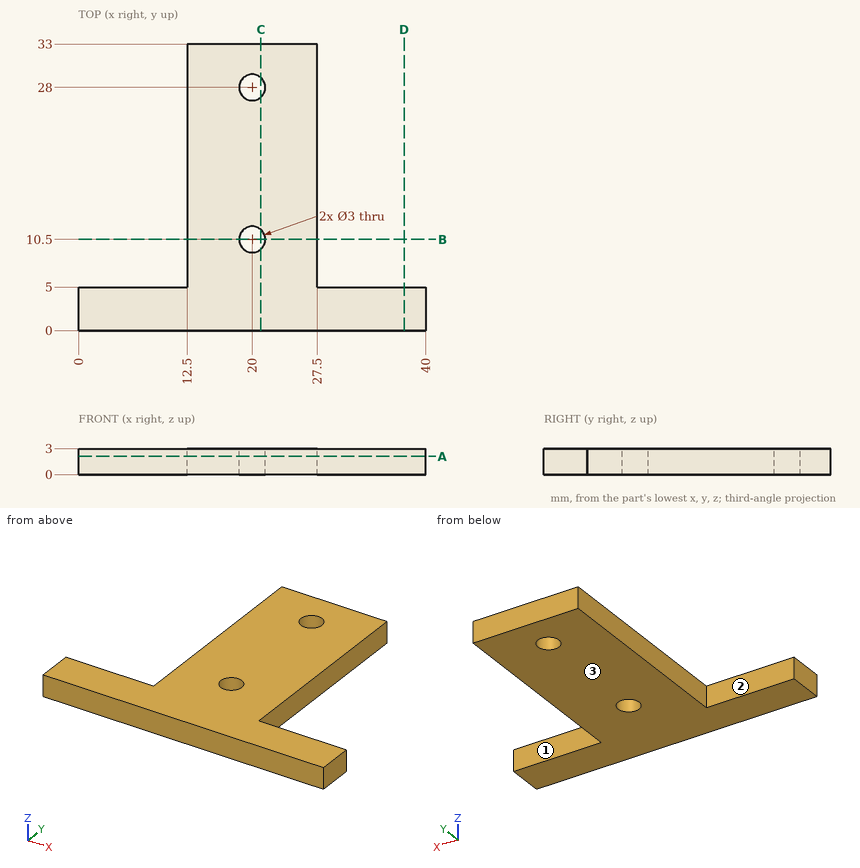
Source: three-view drawing plus pictorial views. Frame: mm from the lowest corner of the part. A direction names the side the tool comes from. Round coordinates to 2 decimals unless told otherwise and drop trailing zeros. Order: outer loops, then holes, each group sorted by start corner. A loop starts at its lowest first (then second) coordinate and runs counter-clockwise, first axis right, second up. Notation, with made-up numbers: (-28, 75) - (-3, 75) arc R7 cw to (-3, 81) - close; hole circle Ø5 at (-21.75, 57.25). An arc over 180 degrees is marked (long way). Use a Markdown table: item, result.
1. First-contact query: pin 1 (0.9 mm diameter, centred on x = 3.5, z = 1, fed in from +Y). Flat tip, straight axial feed; report the tip coordinate or a pass-through.
Evaluation:
| item | result |
|---|---|
| pin 1 | y = 5 |
2. Section C-C on x = 21. Return the cut outline in (y, z), then the cut area to 3 significant figures.
Evaluation:
| item | result |
|---|---|
| outline | (0, 0) - (9.38, 0) - (9.38, 3) - (0, 3) - close; (11.62, 0) - (26.88, 0) - (26.88, 3) - (11.62, 3) - close; (29.12, 0) - (33, 0) - (33, 3) - (29.12, 3) - close |
| area | 85.6 mm^2 |
3. Section A-A on z = 2.1. Return the cut outline in (x, y).
Evaluation:
| item | result |
|---|---|
| outline | (0, 0) - (40, 0) - (40, 5) - (27.5, 5) - (27.5, 33) - (12.5, 33) - (12.5, 5) - (0, 5) - close; hole circle Ø3 at (20, 10.5); hole circle Ø3 at (20, 28) |
4. Material intervals for probe 1 along Y at (x, z) = (20, 0.8); probe 2 along X at (y, z) = (10.5, 2.05); probe 3 along X at (y, z) = (15, 2.75), sorted ascending.
Evaluation:
| item | result |
|---|---|
| probe 1 | 0 to 9, 12 to 26.5, 29.5 to 33 |
| probe 2 | 12.5 to 18.5, 21.5 to 27.5 |
| probe 3 | 12.5 to 27.5 |
5. Access query for the marked faces 1, 2 and 3. Directions: +Z, -Z, +X, -X, +Y, -Y. A direction counts if a zero-diameter tool reaches every point of the face in a straight line with its end or side. Return the directions, or none.
Evaluation:
| item | result |
|---|---|
| face 1 | +Z, -Z, +X, +Y |
| face 2 | +Z, -Z, -X, +Y |
| face 3 | -Z, +X, -X, +Y, -Y |
6. Section B-B on y = 10.5. Return the cut outline in (x, z).
Evaluation:
| item | result |
|---|---|
| outline | (12.5, 0) - (18.5, 0) - (18.5, 3) - (12.5, 3) - close; (21.5, 0) - (27.5, 0) - (27.5, 3) - (21.5, 3) - close |
7. Section D-D on x = 37.5. Return the cut outline in (y, z).
Evaluation:
| item | result |
|---|---|
| outline | (0, 0) - (5, 0) - (5, 3) - (0, 3) - close |
